The listing builds one solid part. Answer for the finished solid, in the listing's coordinates (mm). Face numbers are marked on the shaded views. A direction names the side the tool comes from. Give positions to 0.01 mm unless a question says otherwise; leave off trailing zeros. Write each loop counter-clockwise with the first axis right and the second up, starting at its lowest first coordinate (ties: lowest second). Pieces come first, ordered by that corner, then holes. Notation, with made-up numbers: (61.25, 83) - (102.25, 83) arc R14 ccw to (102.25, 97) - close; hole circle Ø6 at (-27.75, 33.25). An arc over 180 degrees is marked (long way). Answer in a Markdown table with one row per item. Add a question column.
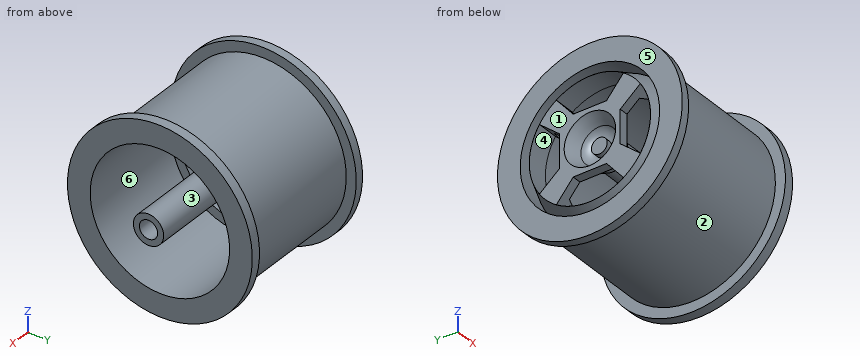
from build123d import *

# Parameters (mm, degrees)
SKETCH4_R           = 1.5
CUT_EXTRUDE1_DEPTH  = 15
CUT_EXTRUDE3_DEPTH  = 15
FILLET1_R           = 2
SKETCH8_R           = 1.305513627
BOSS_EXTRUDE1_DEPTH = 1


with BuildPart() as part:
    # Sketch1 → Revolve1 (revolve)
    with BuildSketch(Plane.XY, mode=Mode.PRIVATE) as revolve1_sk:
        Polygon((0, 15.25), (0, 11.5), (3.6, 11.5), (3.6, 10), (6.6, 10), (6.6, 11.5), (24.65, 11.5), (24.65, 15.25), (23.05, 15.25), (23.05, 13.6), (1.4, 13.6), (1.4, 15.25), align=None)
    revolve(revolve1_sk.sketch.rotate(Axis((0, 0, 0), (1, 0, 0)), 90), axis=Axis((0, 0, 0), (1, 0, 0)))



with BuildPart() as body_2:
    # Sketch3 → Revolve2 (revolve)
    with BuildSketch(Plane.XY, mode=Mode.PRIVATE) as revolve2_sk:
        Polygon((1.5, 0), (27.2, 0), (27.2, 2.5), (5.171947712, 2.5), (1.5, 4.62), align=None)
    revolve(revolve2_sk.sketch.rotate(Axis((0, 0, 0), (1, 0, 0)), 90), axis=Axis((0, 0, 0), (1, 0, 0)))

    # Sketch4 → Cut-Extrude1 (cut)
    with BuildSketch(Plane(origin=(27.2, 0, 0), x_dir=(0, 0, -1), z_dir=(1, 0, 0))):
        Circle(SKETCH4_R)
    extrude(amount=-CUT_EXTRUDE1_DEPTH, mode=Mode.SUBTRACT)


with BuildPart() as part_1:
    add(part.part)

    add(body_2.part)  # Revolve4 merges body 2
    # Sketch5 → Revolve4 (revolve)
    with BuildSketch(Plane.XY):
        Polygon((0, 0), (0, 10), (3.6, 11.5), (3.6, 9.258144762), (1.5, 8.383144762), (1.5, 0), align=None)
    revolve(axis=Axis((1.5, 0, 0), (-1, 0, 0)))

    # Sketch6 → Cut-Extrude3 (cut)
    with BuildSketch(Plane.ZY):
        with BuildLine():
            Line((2.75, 5), (-2.75, 5))
            Line((-2.75, 5), (-5.536071385, 8.320310583))
            ThreePointArc((-5.536071385, 8.320310583), (0, 9.993780795), (5.536071385, 8.320310583))
            Line((5.536071385, 8.320310583), (2.75, 5))
        make_face()
        with BuildLine():
            Line((5, 2.75), (8.320310583, 5.536071385))
            ThreePointArc((8.320310583, 5.536071385), (9.993780795, 0), (8.320310583, -5.536071385))
            Line((8.320310583, -5.536071385), (5, -2.75))
            Line((5, -2.75), (5, 2.75))
        make_face()
        with BuildLine():
            Line((2.75, -5), (5.536071385, -8.320310583))
            ThreePointArc((5.536071385, -8.320310583), (0, -9.993780795), (-5.536071385, -8.320310583))
            Line((-5.536071385, -8.320310583), (-2.75, -5))
            Line((-2.75, -5), (2.75, -5))
        make_face()
        with BuildLine():
            Line((-5, -2.75), (-8.320310583, -5.536071385))
            ThreePointArc((-8.320310583, -5.536071385), (-9.993780795, 0), (-8.320310583, 5.536071385))
            Line((-8.320310583, 5.536071385), (-5, 2.75))
            Line((-5, 2.75), (-5, -2.75))
        make_face()
    extrude(amount=-CUT_EXTRUDE3_DEPTH, mode=Mode.SUBTRACT)

    # Sketch7 → Cut-Revolve1 (revolve, cut)
    with BuildSketch(Plane.XY):
        Polygon((3.1, 0), (0, 0), (0, 4.25), (3.1, 2.460214166), align=None)
    revolve(axis=Axis((3.1, 0, 0), (-1, 0, 0)), mode=Mode.SUBTRACT)

    # Fillet1
    fillet1_edges = [part_1.edges().sort_by_distance(p)[0] for p in [
        (3.1, -2.460214166, 0),
    ]]
    fillet(fillet1_edges, radius=FILLET1_R)

    # Sketch8 → Boss-Extrude1 (add)
    with BuildSketch(Plane.ZY.offset(-3.1)):
        with Locations(Location((0, 0, 0), (0, 0, 270))):
            Circle(SKETCH8_R)
    extrude(amount=BOSS_EXTRUDE1_DEPTH)


solid = part_1.part
1. The mould has two halves that part along Y. Classify the marked faces 1, 2 and 3: +Y half, -Y half, draft (parallel to the pull), parting line (faces both ways), or undercut.
2. Given pin 1 Ø1 at (y, z) = (12, 7.5) entering from +X; pin 2 Ø8 at (x, y) = (8, 8.5) entering from +Z; pin 3 Ø4 at (x, z) = (4, 0.5) entering from +Y, each flat-ended and moving along its own axis, determine where each tip first touches the part or whether it passes through.
3. Straight lines are drawn through the part: L1, parallel to Y at x = 15.75, z = 0; L2, parallel to Y at x = 5.8, z = 0; L3, parallel to Y at x = 11.25, z = 0. For each, find the intervals that lie inside material, in ascending order. Write a range as [from, to].
4. A tool of negligible diameter and unlimited length cuts with its end or side. For the marked faces 4, 5 and 6, from which of +Z, -Z, +X, -X, +Y, -Y can it reach the whole face along a straight path? Write none if from no direction.
5. Section C-C (y = 0) is taken. State how many separate pieces and enclosed holes the cut face has, and give its area (3 significant figures).
6. Section B-B (x = 9) is taken. Give the vertices of the cut face in (y, z), and give its area (3 significant figures).
7. Section A-A (x = 15.5) is taken. Give the vertices of the cut face in (y, z), and give its area (3 significant figures).
Geometry check:
| question | item | result |
|---|---|---|
| 1 | face 1 | draft |
| 1 | face 2 | parting line |
| 1 | face 3 | undercut |
| 2 | pin 1 | x = 24.65 |
| 2 | pin 2 | z = 12.83 |
| 2 | pin 3 | y = 13.6 |
| 3 | L1 | [-13.6, -11.5], [-2.5, -1.5], [1.5, 2.5], [11.5, 13.6] |
| 3 | L2 | [-13.6, -10], [-2.5, 2.5], [10, 13.6] |
| 3 | L3 | [-13.6, -11.5], [-2.5, 2.5], [11.5, 13.6] |
| 4 | face 4 | +X, -X |
| 4 | face 5 | +Z, -Z, -X, +Y, -Y |
| 4 | face 6 | +X |
| 5 | separate pieces | 3 |
| 5 | enclosed holes | 0 |
| 5 | area | 216 mm² |
| 6 | outline | circle Ø27.2 at (0, 0); circle Ø5 at (0, 0); hole circle Ø23 at (0, 0) |
| 6 | area | 185 mm² |
| 7 | outline | circle Ø27.2 at (0, 0); circle Ø5 at (0, 0); hole circle Ø23 at (0, 0); hole circle Ø3 at (0, 0) |
| 7 | area | 178 mm² |
